Work out the finished part from the listing and answer in its coordinate system (mm). Round coordinates to 2 decimals unless told otherwise and drop trailing zeros. Write each loop counter-clockwise with the first axis right and the second up, starting at its lowest first coordinate (ties: lowest second). Pieces come first, ordered by that corner, then holes.
from build123d import *

# Parameters (mm, degrees)
F1_DEPTH = 5


with BuildPart() as f1:
    # F0 (on Front) → F1 (new body)
    with BuildSketch(Plane.XZ):
        with BuildLine():
            ThreePointArc((39.671052, -35.230264), (52.427442, -19.776479), (55.657893, 0))
            ThreePointArc((55.657893, 0), (27.828947, 27.828947), (0, 0))
            ThreePointArc((0, 0), (-7.19782, 16.589503), (-22.607862, 26.052631))
            ThreePointArc((-22.607862, 26.052631), (-42.123539, 18.190011), (-52.697372, 0))
            ThreePointArc((-52.697372, 0), (-52.395006, -19.601983), (-40.559214, -35.230264))
            Line((-40.559214, -35.230264), (0, -63.351638))
            Line((0, -63.351638), (39.671052, -35.230264))
        make_face()
    extrude(amount=F1_DEPTH)


solid = f1.part
Q1. The mould has two halves that part along X. Classify faces 1 (the face through (-7.03, -2.465, 16.395)), 2 (the face through (-52.485, -2.465, -19.338)), 3 (the face through (0, -5, -17)): +X half, -X half, draft (parallel to the pull), parting line (faces both ways), or undercut.
Q2. Find section B-B (z = 4.5). Determine the outline of the cut face in (x, y), plus the area to 3 significant figures.
Q3. Find the intervals of material crossed by L1, parallel to X at y = -2.15, z = 18; L2, parallel to X at y = -2.3, z = 17; L3, parallel to Z at x = 18, y = -0.8, in increasing order.
Q4. Given pin 1 (1.5 mm diameter, centred on x = 32.5, y = -1.5, fed in from -Z); pin 2 (1.5 mm diameter, centred on x = -23.5, y = -2, fed in from -Z), each flat-ended and moving along its own axis, determine where each tip first touches the part or whether it passes through.
Q5. Find section D-D (z = -51). Determine the outline of the cut face in (x, y).
Q6. Find section C-C (x = 17). Determine the outline of the cut face in (y, z).
Q7. Find section A-A (y = -3.7). Determine the outline of the cut face in (x, z).
Report:
1. face 1: undercut
1. face 2: -X half
1. face 3: draft
2. outline: (-51.46, -5) - (-0.82, -5) - (-0.82, 0) - (-51.46, 0) - close; (0.37, -5) - (55.29, -5) - (55.29, 0) - (0.37, 0) - close
2. area: 528 mm2
3. L1: x = -42.34 to -8.5, 6.61 to 49.05
3. L2: x = -43.42 to -7.56, 5.8 to 49.86
3. L3: z = -50.59 to 26.04
4. pin 1: stops at z = -40.85
4. pin 2: stops at z = -47.58
5. outline: (-17.81, -5) - (17.42, -5) - (17.42, 0) - (-17.81, 0) - close
6. outline: (-5, -51.3) - (0, -51.3) - (0, 25.64) - (-5, 25.64) - close
7. outline: (-52.7, 0) arc R31.51 ccw to (-40.56, -35.23) - (0, -63.35) - (39.67, -35.23) arc R38.39 ccw to (55.66, 0) arc R27.83 ccw to (0, 0) arc R30.08 ccw to (-22.61, 26.05) arc R32.41 ccw to start
